Geometry check sheet. Reference: the model listing, model coordinates, mm. A direction names the side the tool comes from. Round coordinates to 2 decimals unless told otherwise and drop trailing zeros. Order: outer loops, then holes, each group sorted by start corner. A loop starts at its lowest first (then second) coordinate and runs counter-clockwise, first axis right, second up. Notation, with made-up numbers: (72, 42) - (85, 42) arc R22 ccw to (85, 60) - close; hole circle Ø8 at (-10.5, 29). An arc over 180 degrees is marked (long way). Write each question's results on one line, items separated by ' | '.
```python
from build123d import *

# Parameters (mm, degrees)
BOSS_EXTRUDE1_DEPTH             = 3.175
F_1_4_0_25_DIAMETER_HOLE1_D     = 6.35
F_1_4_0_25_DIAMETER_HOLE1_DEPTH = 9.268267535
F_1_4_0_25_DIAMETER_HOLE1_TIP   = 1.907732465
FILLET1_R                       = 12.7


with BuildPart() as part:
    # Sketch1 → Boss-Extrude1 (new body)
    with BuildSketch(Plane.XY):
        with BuildLine():
            Line((427.919423357, 0), (440.619423357, 0))
            Line((440.619423357, 0), (461.846041333, -16.2036647))
            ThreePointArc((461.846041333, -16.2036647), (463.98221908, -31.261387982), (450.144423357, -37.571197432))
            Line((450.144423357, -37.571197432), (427.919423357, -25.4))
            Line((427.919423357, -25.4), (427.919423357, -22.225))
            Line((427.919423357, -22.225), (424.744423357, -22.225))
            Line((424.744423357, -22.225), (424.744423357, -3.175))
            Line((424.744423357, -3.175), (427.919423357, -3.175))
            Line((427.919423357, -3.175), (427.919423357, 0))
        make_face()
    extrude(amount=BOSS_EXTRUDE1_DEPTH)

    # 1/4 (0.25) Diameter Hole1
    with Locations(Plane.XY.offset(3.175)):
        with Locations((452.843173357, -25.161251887)):
            Hole(F_1_4_0_25_DIAMETER_HOLE1_D / 2, depth=F_1_4_0_25_DIAMETER_HOLE1_DEPTH)
            with Locations((0, 0, -(F_1_4_0_25_DIAMETER_HOLE1_DEPTH + F_1_4_0_25_DIAMETER_HOLE1_TIP / 2))):  # 118° drill point
                Cone(0, F_1_4_0_25_DIAMETER_HOLE1_D / 2, F_1_4_0_25_DIAMETER_HOLE1_TIP, mode=Mode.SUBTRACT)

    # Fillet1
    fillet1_edges = [part.edges().sort_by_distance(p)[0] for p in [
        (440.619423357, 0, 1.5875),
    ]]
    fillet(fillet1_edges, radius=FILLET1_R)


solid = part.part
```
(1) Material ranges on line 1 (X direction, y = -28, z = 0.7); line 2 (X direction, y = -22.5, z = 1.85); line 3 (Y direction, x = 454, z = 2), recorded low to high.
Answers follow:
line 1: 432.67 to 451.42, 454.27 to 465.22 | line 2: 427.92 to 451.11, 454.57 to 465.26 | line 3: -37.81 to -28.12, -22.2 to -10.21
(2) Depth check by flat-ended pin: pin 1 Ø1 at (y, z) = (-23.5, 1.5) entering from -X; pin 2 Ø1.5 at (y, z) = (-30, 1) entering from +X. Enter the tip coordinate at first touch or a pass-through.
Answers follow:
pin 1: x = 427.92 | pin 2: x = 464.87
(3) Section check A-A (y = -27). Record the cut outline in (x, z) (3 decimals), then the cut area to 3 significant figures.
Answers follow:
outline: (430.841, 0) - (450.255, 0) - (450.255, 3.175) - (430.841, 3.175) - close; (455.432, 0) - (465.409, 0) - (465.409, 3.175) - (455.432, 3.175) - close | area: 93.3 mm²
(4) Access from +Z, -Z, +X, -X, +Y, -Y to the whole of each face (thin tool, end or side, straight path). Record for faces 4 (the face through (426, -22.225, 2)), 5 (the face through (445, -19, 3.175)), 6 (the face through (426, -3.175, 2)).
Answers follow:
face 4: +Z, -Z, -X, -Y | face 5: +Z, +X, -X, +Y, -Y | face 6: +Z, -Z, -X, +Y
(5) Section check D-D (x = 427). Record the cut outline in (y, z) (3 decimals).
Answers follow:
outline: (-22.225, 0) - (-3.175, 0) - (-3.175, 3.175) - (-22.225, 3.175) - close
(6) Section check C-C (x = 454). Record the cut outline in (y, z) (1 decimal).
Answers follow:
outline: (-37.8, 0) - (-28.1, 0) - (-28.1, 3.2) - (-37.8, 3.2) - close; (-22.2, 0) - (-10.2, 0) - (-10.2, 3.2) - (-22.2, 3.2) - close
(7) Section check B-B (z = 2.4). Record the cut outline in (x, y) (3 decimals), then the cut area to 3 significant figures.
Answers follow:
outline: (424.744, -22.225) - (427.919, -22.225) - (427.919, -25.4) - (450.144, -37.571) arc R12.7 ccw to (461.846, -16.204) - (444.032, -2.605) arc R12.7 ccw to (436.326, 0) - (427.919, 0) - (427.919, -3.175) - (424.744, -3.175) - close; hole circle Ø6.35 at (452.843, -25.161) | area: 1,030 mm²
(8) Draft check along X on faces 1 (the face through (445, -19, 0)), 2 (the face through (449.815, -24.208, 1.565)), 3 (the face through (427.919, -24, 2)). Enter one of: released by +X, released by -X, zero draft, split by the parting line, or undercut.
Answers follow:
face 1: zero draft | face 2: undercut | face 3: released by -X
